from build123d import *

# Parameters (mm, degrees)
SKETCH_1_R          = 6.5
SKETCH_1_R_2        = 4.05
SKETCH_1_R_3        = 1.55
EXTRUDE_1_DEPTH     = 5
FILLET_1_R          = 40
CUT_EXTRUDE_1_DEPTH = 160.010002676


with BuildPart() as part:
    # 草图1 → 凸台-拉伸1 (new body)
    # profile 1 of 5: a face of its own
    with BuildSketch(Plane.XY):
        Circle(SKETCH_1_R)
        Circle(SKETCH_1_R_2, mode=Mode.SUBTRACT)
    # profile 2 of 5: a face of its own
    with BuildSketch(Plane.XY):
        with BuildLine():
            ThreePointArc((6.5, 0), (5.051052449, -4.091071884), (1.350194104, -6.358221126))
            Line((1.350194104, -6.358221126), (55.199071912, 5.076806988))
            ThreePointArc((55.199071912, 5.076806988), (48.73376571, 10.906123973), (53.864865433, 17.938402155))
            Line((53.864865433, 17.938402155), (-1.334206479, 6.361595167))
            ThreePointArc((-1.334206479, 6.361595167), (4.09741735, 5.045906366), (6.5, 0))
        make_face()
    # profile 3 of 5: a face of its own
    with BuildSketch(Plane.XY):
        with Locations((55.199071912, 11.576806988)):
            Circle(SKETCH_1_R)
        with Locations((55.199071912, 11.576806988)):
            Circle(SKETCH_1_R_3, mode=Mode.SUBTRACT)
    # profile 4 of 5: a face of its own
    with BuildSketch(Plane.XY):
        with BuildLine():
            ThreePointArc((61.699071912, 11.576806988), (59.79526599, 6.98061291), (55.199071912, 5.076806988))
            Line((55.199071912, 5.076806988), (150.620267879, -6.45306267))
            ThreePointArc((150.620267879, -6.45306267), (144.946748663, 0.778169119), (152.176606073, 6.453439626))
            Line((152.176606073, 6.453439626), (55.975677985, 18.030246614))
            ThreePointArc((55.975677985, 18.030246614), (60.062092551, 15.88969816), (61.699071912, 11.576806988))
        make_face()
    # profile 5 of 5: a face of its own
    with BuildSketch(Plane.XY):
        with Locations((151.4, 0)):
            Circle(SKETCH_1_R)
        with Locations((151.4, 0)):
            Circle(SKETCH_1_R_3, mode=Mode.SUBTRACT)
    extrude(amount=EXTRUDE_1_DEPTH)

    # 圆角1
    fillet_1_edges = [part.edges().sort_by_distance(p)[0] for p in [
        (55.199071912, 5.076806988, 2.5),
    ]]
    fillet(fillet_1_edges, radius=FILLET_1_R)

    # 草图2 → 切除-拉伸1 (cut, through all)
    with BuildSketch(Plane.XY.offset(5)):
        with BuildLine():
            Line((71.442895333, 12.643671867), (135.873043723, 4.890156314))
            ThreePointArc((135.873043723, 4.890156314), (138.493120748, 1.553212146), (135.156176579, -1.066864879))
            Line((135.156176579, -1.066864879), (70.726028189, 6.686650674))
            ThreePointArc((70.726028189, 6.686650674), (68.105951164, 10.023594842), (71.442895333, 12.643671867))
        make_face()
    extrude(amount=-CUT_EXTRUDE_1_DEPTH, mode=Mode.SUBTRACT)


solid = part.part
For this review, take the finished solid that the model builds, in its own axes (mm). A direction names the side the tool comes from. Give positions to 0.01 mm unless a question says otherwise; leave off trailing zeros. Order: outer loops, then holes, each group sorted by start corner. A loop starts at its lowest first (then second) coordinate and runs counter-clockwise, first axis right, second up. Notation, with made-up numbers: M 61.25,-19 L 73.25,-19 A22 ccw 73.25,-4 Z; hole C 7.5,69 d6. An arc over 180 degrees is marked long. Answer in a Markdown table with one row per item. Add a question column.
(1) Wall thickness on probe 1 along Y at (x, z) = (102.5, 4.5); probe 2 along Y at (x, z) = (95, 1.9); probe 3 along Y at (x, z) = (143, 2.7): over which ranges is each line inside the solid? List them lowest first. Write a range as [from, to].
(2) Consider section D-D on x = 30. State the section outline as (y, z) points, and give its area (3 significant figures).
(3) Consider section B-B on z = 1.05. State the section outline as (x, y) points, and give its area (3 significant figures).
(4) Consider section A-A on x = 87.5. State the section outline as (y, z) points.
(5) For pin 1 (1.5 mm diameter, centred on x = 66.5, z = 3, fed in from +Y); pin 2 (1 mm diameter, centred on x = 29, z = 2.5, fed in from +Y); pin 3 (1 mm diameter, centred on x = 102.5, z = 4.5, fed in from -Y), all flat-tipped, find the tip position at first contact; note any pin that passes through.
(6) Mouldability with a two-part tool opening along Y and no side actions: class faces 1 (the face through (75, 6, 0)), 2 (the face through (68.1, 9.96, 2.54)), 3 (the face through (24.7, -1.4, 2.5)) as +Y half, -Y half, draft (parallel to the pull), parting line (faces both ways), or undercut.
(7) Consider section C-C on x = 0. State the section outline as (y, z) points, and give its area (3 significant figures).
(8) For faces 4 (the face through (103.392, 2.756, 2.535)), 5 (the face through (105.59, -1.01, 2.46)), 6 (the face through (26.65, 12.23, 2.46)), list the 3-axis set-ups (+Z, -Z, +X, -X, +Y, -Y) from which the entire face can be reached by the end or side of a thin tool; tool diameter is ignored.
Evaluation:
| question | item | result |
|---|---|---|
| 1 | probe 1 | y = [-0.64, 2.86], [8.91, 12.43] |
| 1 | probe 2 | y = [0.27, 3.77], [9.81, 13.33] |
| 1 | probe 3 | y = [-5.53, 7.56] |
| 2 | outline | M -0.27,0 L 12.93,0 L 12.93,5 L -0.27,5 Z |
| 2 | area | 66.0 mm^2 |
| 3 | outline | M -1.33,6.36 A6.5 ccw 1.35,-6.36 L 48.69,3.7 A40 cw 61.8,4.28 L 150.62,-6.45 A6.5 ccw 152.18,6.45 L 55.98,18.03 A6.5 ccw 53.86,17.94 Z; hole C 0,0 d8.1; hole C 55.2,11.58 d3.1; hole M 70.73,6.69 L 135.16,-1.07 A3 ccw 135.87,4.89 L 71.44,12.64 A3 ccw Z; hole C 151.4,0 d3.1 |
| 3 | area | 1,640 mm^2 |
| 4 | outline | M 1.17,0 L 4.67,0 L 4.67,5 L 1.17,5 Z; M 10.71,0 L 14.24,0 L 14.24,5 L 10.71,5 Z |
| 5 | pin 1 | stops at y = 16.85 |
| 5 | pin 2 | stops at y = 12.83 |
| 5 | pin 3 | stops at y = -0.7 |
| 6 | face 1 | draft |
| 6 | face 2 | undercut |
| 6 | face 3 | -Y half |
| 7 | outline | M -6.5,0 L -4.05,0 L -4.05,5 L -6.5,5 Z; M 4.05,0 L 6.64,0 L 6.64,5 L 4.05,5 Z |
| 7 | area | 25.2 mm^2 |
| 8 | face 4 | +Z, -Z |
| 8 | face 5 | +Z, -Z, -Y |
| 8 | face 6 | +Z, -Z, -X, +Y |
